from build123d import *

# Parameters (mm, degrees)
SKETCH1_R              = 25.527
BOARD_DEPTH            = 1.6
SKETCH2_R              = 1.13
NON_PLATED_HOLES_DEPTH = 76.630682782


with BuildPart() as part:
    # Sketch1 → BOARD (new body)
    with BuildSketch(Plane.XY):
        with Locations((27.94, 27.94)):
            Circle(SKETCH1_R)
    extrude(amount=BOARD_DEPTH)

    # Sketch2 → NON-PLATED HOLES (cut, through all)
    with BuildSketch(Plane.XY):
        with Locations((48.64, 39.5)):
            Circle(SKETCH2_R)
        with Locations((48.64, 16.38)):
            Circle(SKETCH2_R)
        with Locations((16.89, 39.5)):
            Circle(SKETCH2_R)
        with Locations((16.89, 16.38)):
            Circle(SKETCH2_R)
    extrude(amount=NON_PLATED_HOLES_DEPTH, mode=Mode.SUBTRACT)


solid = part.part
Geometry check sheet. Reference: the model listing, model coordinates, mm. Give positions to 0.01 mm unless a question says otherwise; leave off trailing zeros. Order: outer loops, then holes, each group sorted by start corner. A loop starts at its lowest first (then second) coordinate and runs counter-clockwise, first axis right, second up.
1. Sectioned sample at A-A (x = 48.64). Record the boundary of the cut face in (y, z).
Completed:
outline: (13, 0) - (15.25, 0) - (15.25, 1.6) - (13, 1.6) - close; (17.51, 0) - (38.37, 0) - (38.37, 1.6) - (17.51, 1.6) - close; (40.63, 0) - (42.88, 0) - (42.88, 1.6) - (40.63, 1.6) - close
2. Draft check along Y on faces 1 (the face through (47.51, 16.43, 0.79)), 2 (the face through (24.62, 53.25, 0.79)), 3 (the face through (28, 28, 0)). Enter one of: pulls with the +Y half, pulls with the -Y half, needs draft (parallel to the pull), parting line crosses it, or undercut.
Completed:
face 1: undercut
face 2: parting line crosses it
face 3: needs draft
3. Depth check by flat-ended pin: pin 1 (1.8 mm diameter, centred on x = 48.64, y = 16.38, fed in from +Z). Enter the tip coordinate at first touch or a pass-through.
Completed:
pin 1: passes through
4. Scan lines: line 1 (Y direction, x = 48.64, z = 1.25); line 2 (Y direction, x = 16.89, z = 0.5); line 3 (X direction, y = 16.38, z = 0.65). Record each from-to range of solid material in increasing order.
Completed:
line 1: y = 13 to 15.25, 17.51 to 38.37, 40.63 to 42.88
line 2: y = 4.93 to 15.25, 17.51 to 38.37, 40.63 to 50.95
line 3: x = 5.18 to 15.76, 18.02 to 47.51, 49.77 to 50.7
5. Sectioned sample at D-D (y = 37). Record the boundary of the cut face in (x, z), then the cut area to 3 significant figures.
Completed:
outline: (4.07, 0) - (51.81, 0) - (51.81, 1.6) - (4.07, 1.6) - close
area: 76.4 mm2
6. Sectioned sample at B-B (z = 0.65). Record the boundary of the cut face in (x, y).
Completed:
outline: circle Ø51.05 at (27.94, 27.94); hole circle Ø2.26 at (16.89, 16.38); hole circle Ø2.26 at (16.89, 39.5); hole circle Ø2.26 at (48.64, 16.38); hole circle Ø2.26 at (48.64, 39.5)
7. Sectioned sample at C-C (y = 16.38). Record the boundary of the cut face in (x, z).
Completed:
outline: (5.18, 0) - (15.76, 0) - (15.76, 1.6) - (5.18, 1.6) - close; (18.02, 0) - (47.51, 0) - (47.51, 1.6) - (18.02, 1.6) - close; (49.77, 0) - (50.7, 0) - (50.7, 1.6) - (49.77, 1.6) - close
